The drawing under review shows one solid part. Ordinate dimensions are in mm from its lowest x, y, z. A direction names the side the tool comes from. Coordinates: 2 decimals unless noted, no trailing zeros. Order: outer loops, then holes, each group sorted by start corner. A loop starts at its lowest first (then second) coordinate and runs counter-clockwise, first axis right, second up. Notation, with made-up numbers: (-6, -8.5) -> (3, -8.5) arc R4 ccw to (3, -2.5) -> close; hole circle Ø2 at (4.25, 17.5). An arc over 180 degrees is marked (long way). Put each result on its own line as item: value.
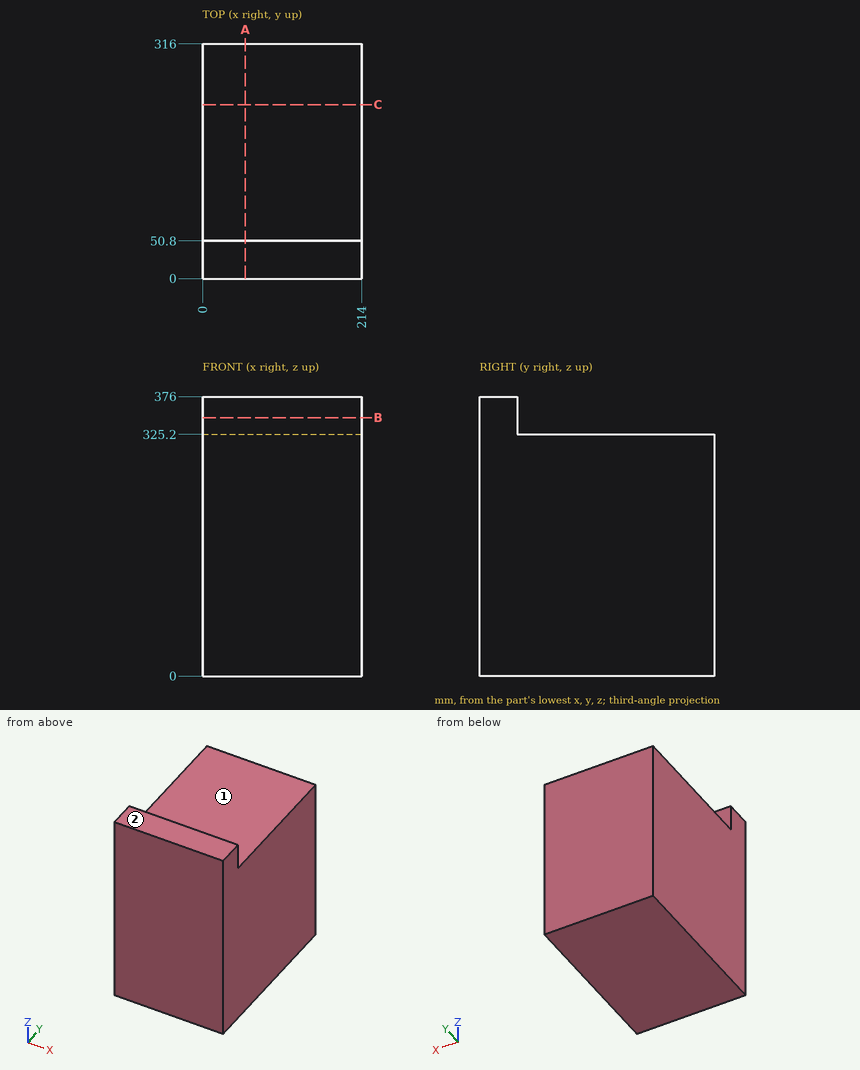
Item 1: Consider section A-A on x = 57.5. Write out the cut boundary in (y, z), and give its area (3 significant figures).
Answers below:
outline: (0, 0) -> (316, 0) -> (316, 325.2) -> (50.8, 325.2) -> (50.8, 376) -> (0, 376) -> close
area: 105,000 mm^2
Item 2: For the marked faces 1 and 2, list the 3-axis set-ups (+Z, -Z, +X, -X, +Y, -Y) from which the entire face can be reached by the end or side of a thin tool; tool diameter is ignored.
Answers below:
face 1: +Z, +X, -X, +Y
face 2: +Z, +X, -X, +Y, -Y
Item 3: Consider section C-C on y = 234.5. Write out the cut boundary in (x, z).
Answers below:
outline: (0, 0) -> (214, 0) -> (214, 325.2) -> (0, 325.2) -> close
Item 4: For pin 1 Ø10 at (x, y) = (187.5, 194) entering from +Z; pin 2 Ø15 at (x, z) = (102.5, 352.5) entering from +Y, all flat-tipped, find the tip position at first contact; note any pin that passes through.
Answers below:
pin 1: z = 325.2
pin 2: y = 50.8
Item 5: Consider section B-B on z = 348. Write out the cut boundary in (x, y).
Answers below:
outline: (0, 0) -> (214, 0) -> (214, 50.8) -> (0, 50.8) -> close
Item 6: For line 1 (Z direction, x = 114.5, y = 182); line 2 (Y direction, x = 80, z = 328), list the stretches that pass through material, from the lowest coordinate up. Write a range as from..to.
Answers below:
line 1: 0..325.2
line 2: 0..50.8
